from build123d import *

# Parameters (mm, degrees)
BOSS_EXTRUDE1_DEPTH = 23.0124
SKETCH2_W           = 44.611940252
SKETCH2_H           = 41.110401543
SKETCH2_R           = 11.5062
CUT_EXTRUDE3_DEPTH  = 2.54
SKETCH3_R           = 3.175
CUT_EXTRUDE4_DEPTH  = 2.408910713


with BuildPart() as part:
    # Sketch1 → Boss-Extrude1 (new body)
    with BuildSketch(Plane.XY):
        with BuildLine():
            Line((-11.5062, -46.279589387), (11.5062, -46.279589387))
            ThreePointArc((11.5062, -46.279589387), (0, -47.6885), (-11.5062, -46.279589387))
        make_face()
    extrude(amount=BOSS_EXTRUDE1_DEPTH)

    # Sketch2 → Cut-Extrude3 (cut)
    with BuildSketch(Plane(origin=(0, -46.279589387, 0), x_dir=(1, 0, 0), z_dir=(0, 1, 0))):
        with Locations((2.111795661, -11.044209065)):
            Rectangle(SKETCH2_W, SKETCH2_H)
        with Locations((0, -11.5062)):
            Circle(SKETCH2_R, mode=Mode.SUBTRACT)
    extrude(amount=-CUT_EXTRUDE3_DEPTH, mode=Mode.SUBTRACT)

    # Sketch3 → Cut-Extrude4 (cut, through all)
    with BuildSketch(Plane(origin=(0, -46.279589387, 0), x_dir=(1, 0, 0), z_dir=(0, 1, 0))):
        with Locations((0, -11.5062)):
            Circle(SKETCH3_R)
    extrude(amount=-CUT_EXTRUDE4_DEPTH, mode=Mode.SUBTRACT)


solid = part.part
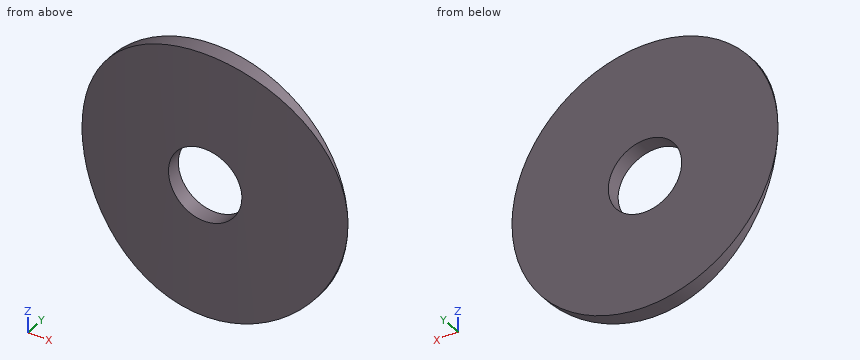
The listing builds one solid part. Answer for the finished solid, in the listing's coordinates (mm). Coordinates: 2 decimals unless noted, no trailing zeros. Order: outer loops, then holes, each group sorted by start corner. A loop starts at its lowest first (then second) coordinate and runs counter-clockwise, first axis right, second up. Notation, with made-up numbers: (30.25, 63.25) -> (59.25, 63.25) arc R24 ccw to (59.25, 90.25) -> close; hole circle Ø1 at (-1, 32). An arc over 180 degrees is marked (long way). Answer in a Markdown table with one row per item. Add a question column.
Item 1: Each of these flat-tipped pins is pushed along its axis until it touches: P1, Ø3, axis at x = -4.5, z = 12.5, coming from the -Y side; P2, Ø4, axis at x = 0, z = 11.51, coming from the -Y side. Where does it stop, or does it pass through?
Item 2: Find section B-B (z = 9). Write down the section's boundary in (x, y), then the cut area to 3 significant figures.
Item 3: Find section A-A (x = 0). Write down the section's boundary in (y, z).
Item 4: Find the intervals of material crossed by L1, parallel to Z at x = 0, y = -46.75; L2, parallel to X at y = -46.8, z = 20.5; L3, parallel to Y at x = -5.5, z = 18, in increasing order. Write a range as from..to.
Item 5: Find section C-C (z = 21.25). Write down the section's boundary in (x, y), then the cut area to 3 significant figures.
Item 6: Find section D-D (x = 3.75). Write down the section's boundary in (y, z), then the cut area to 3 significant figures.
Result set:
| question | item | result |
|---|---|---|
| 1 | P1 | stops at y = -47.59 |
| 1 | P2 | passes through |
| 2 | outline | (-11.23, -46.35) arc R47.69 ccw to (-1.95, -47.65) -> (-1.95, -46.28) -> (-11.23, -46.28) -> close; (1.95, -47.65) arc R47.69 ccw to (11.23, -46.35) -> (11.23, -46.28) -> (1.95, -46.28) -> close |
| 2 | area | 16.2 mm² |
| 3 | outline | (-47.69, 0) -> (-46.28, 0) -> (-46.28, 8.33) -> (-47.69, 8.33) -> close; (-47.69, 14.68) -> (-46.28, 14.68) -> (-46.28, 23.01) -> (-47.69, 23.01) -> close |
| 4 | L1 | z = 0..8.33, 14.68..23.01 |
| 4 | L2 | x = -7.18..7.18 |
| 4 | L3 | y = -47.37..-46.28 |
| 5 | outline | (-6.12, -47.29) arc R47.69 ccw to (6.12, -47.29) -> (6.12, -46.28) -> (-6.12, -46.28) -> close |
| 5 | area | 15.6 mm² |
| 6 | outline | (-47.54, 0.63) -> (-46.28, 0.63) -> (-46.28, 22.38) -> (-47.54, 22.38) -> close |
| 6 | area | 27.4 mm² |
